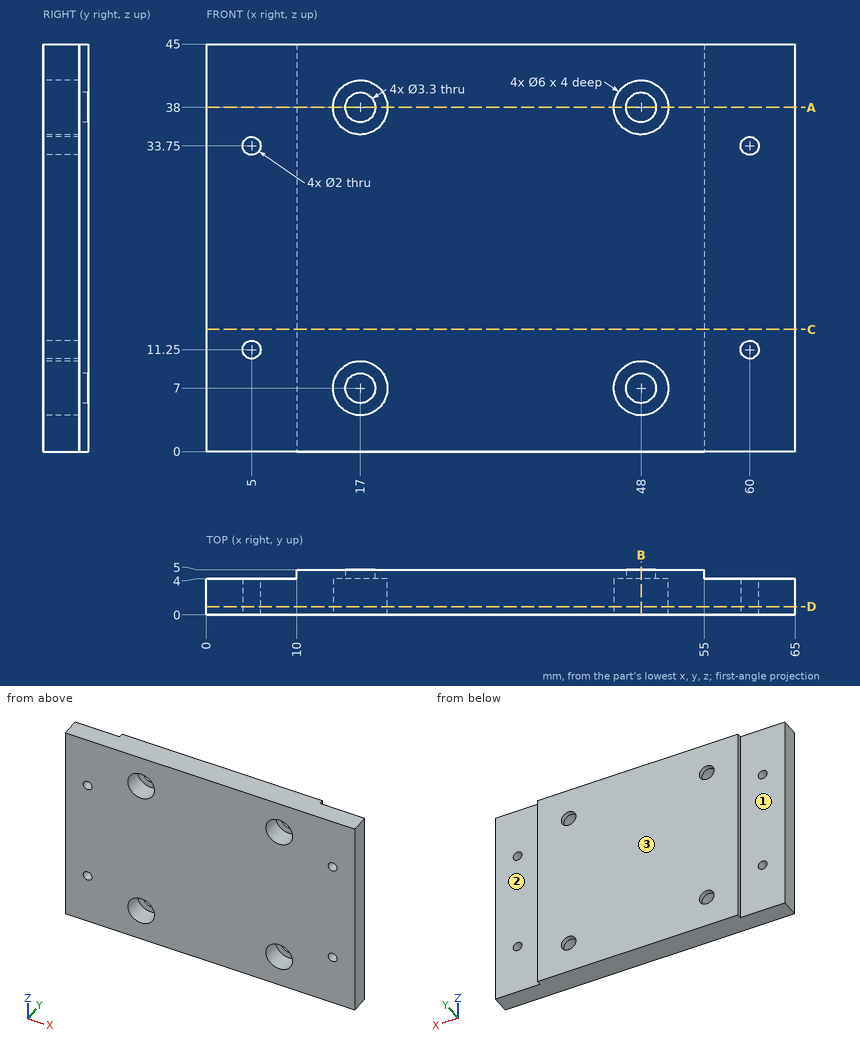
Verification items for this drawing (mm, ordinates from the low corner). A direction names the side the tool comes from. Give positions to 0.01 mm unless a question says otherwise; leave off trailing zeros. Write each loop counter-clockwise with the first axis right and the second up, starting at its lowest first coordinate (ties: lowest second). Pieces come first, ordered by that corner, then holes. Notation, with made-up numbers: (14, 50) - (65, 50) arc R24 ccw to (65, 70) - close; hole circle Ø8 at (27.25, 26). An arc over 180 degrees is marked (long way). Answer as a JSON object with one key per item and string values. Group by question number.
1) Access from +Z, -Z, +X, -X, +Y, -Y to the whole of each face (thin tool, end or side, straight path). Record for the marked faces 1, 2 and 3.
2) Sectioned sample at D-D (y = 0.9). Give the number of separate pieces and of enclosed holes in the cut face, then the cut area to 3 significant figures.
3) Thickness scan on probe 1 along Z at (x, y) = (5, 2.4); probe 2 along Z at (x, y) = (17, 4.7); probe 3 along X at (y, z) = (1.9, 7). Record the ranges inside material, lowest first. Write a range as from..to.
4) Sectioned sample at A-A (z = 38). Record the cut outline in (x, y).
5) Sectioned sample at B-B (x = 48). Record the cut outline in (y, z).
6) Sectioned sample at C-C (z = 13.5). Record the cut outline in (x, y).
7) Depth check by flat-ended pin: P1, Ø2.5, axis at x = 5, z = 33.75, coming from the +Y side; P2, Ø1.8, axis at x = 60, z = 11.25, coming from the +Y side; P3, Ø4.5, axis at x = 17, z = 38, coming from the -Y side. Enter the tip coordinate at first touch or a pass-through.
Geometry results:
{
 "1": {"face 1": "+Z, -Z, -X, +Y", "face 2": "+Z, -Z, +X, +Y", "face 3": "+Z, -Z, +X, -X, +Y"},
 "2": {"separate pieces": "1", "enclosed holes": "8", "area": "2,800 mm^2"},
 "3": {"probe 1": "z = 0..10.25, 12.25..32.75, 34.75..45", "probe 2": "z = 0..5.35, 8.65..36.35, 39.65..45", "probe 3": "x = 0..14, 20..45, 51..65"},
 "4": {"outline": "(0, 0) - (14, 0) - (14, 4) - (15.35, 4) - (15.35, 5) - (10, 5) - (10, 4) - (0, 4) - close; (18.65, 4) - (20, 4) - (20, 0) - (45, 0) - (45, 4) - (46.35, 4) - (46.35, 5) - (18.65, 5) - close; (49.65, 4) - (51, 4) - (51, 0) - (65, 0) - (65, 4) - (55, 4) - (55, 5) - (49.65, 5) - close"},
 "5": {"outline": "(0, 0) - (5, 0) - (5, 5.35) - (4, 5.35) - (4, 4) - (0, 4) - close; (0, 10) - (4, 10) - (4, 8.65) - (5, 8.65) - (5, 36.35) - (4, 36.35) - (4, 35) - (0, 35) - close; (0, 41) - (4, 41) - (4, 39.65) - (5, 39.65) - (5, 45) - (0, 45) - close"},
 "6": {"outline": "(0, 0) - (65, 0) - (65, 4) - (55, 4) - (55, 5) - (10, 5) - (10, 4) - (0, 4) - close"},
 "7": {"P1": "stops at y = 4", "P2": "passes through", "P3": "stops at y = 4"}
}
